```python
from build123d import *

# Parameters (mm, degrees)
F0_W     = 38.1
F0_H     = 25.4
F1_DEPTH = 50.8
F2_D     = 76.2


with BuildPart() as f1:
    # F0 (on Front) → F1 (new body)
    with BuildSketch(Plane.XZ):
        with BuildLine():
            ThreePointArc((0, 103.7758213215), (-54.7329493961, 81.9335598316), (-77.5202206336, 27.5872590731))
            Line((-77.5202206336, 27.5872590731), (-1.3202206336, 27.5872590731))
            Line((-1.3202206336, 27.5872590731), (0, 103.7758213215))
        make_face()
        Polygon((-1.3202206336, 27.5872590731), (-77.5202206336, 27.5872590731), (-77.5202206336, -43.5327409269), (-39.4202206336, -43.5327409269), (36.7797793664, -43.5327409269), (74.8797793664, -43.5327409269), (74.8797793664, 27.5872590731), align=None)
        with BuildLine():
            Line((0, 103.7758213215), (-1.3202206336, 27.5872590731))
            Line((-1.3202206336, 27.5872590731), (74.8797793664, 27.5872590731))
            ThreePointArc((74.8797793664, 27.5872590731), (53.026080125, 80.9999878356), (0, 103.7758213215))
        make_face()
        with Locations((-58.4702206336, -56.2327409269)):
            Rectangle(F0_W, F0_H)
        with Locations((55.8297793664, -56.2327409269)):
            Rectangle(F0_W, F0_H)
    extrude(amount=F1_DEPTH)

    # F2 (through all)
    with Locations(Plane(origin=(0, 0, 0), x_dir=(1, 0, 0), z_dir=(0, 1, 0))):
        with Locations((-1.3202206336, -27.5872590731)):
            Hole(F2_D / 2)


solid = f1.part
```
Could you check a few things on this model? Use its own coordinates, in mm. A direction names the side the tool comes from. Give positions to 0.01 mm unless a question says otherwise; leave off trailing zeros. Loops run counter-clockwise (first coordinate to the right, second up) from the corner with the lowest first, then second, coordinate; pieces in that order, holes last. Notation, with made-up numbers: (6.25, 65) -> (54.25, 65) arc R15 ccw to (54.25, 92) -> close; hole circle Ø4 at (67, -15.5). An arc over 180 degrees is marked (long way). Put each result on its own line as item: value.
(1) Imagine slicing it at D-D on x = 57. Write out the boundary of the cut face in (y, z).
Computed:
outline: (-50.8, -68.93) -> (0, -68.93) -> (0, 76.63) -> (-50.8, 76.63) -> close
(2) Thinking about a two-plate mould opening in X: for faces 3 (the face through (-59, -25, -68.933)), 4 (the face through (-2, -25, -43.533)), 5 (the face through (6.94, -25.76, 64.78)), 6 (the face through (74.88, -25, -21)), which applies, pulls with the +X half, pulls with the -X half, needs draft (parallel to the pull), parting line crosses it, or undercut?
Computed:
face 3: needs draft
face 4: undercut
face 5: undercut
face 6: pulls with the +X half
(3) Imagine slicing it at C-C on z = 63.5. Write out the boundary of the cut face in (x, y), plus the area to 3 significant figures.
Computed:
outline: (-68.53, -50.8) -> (-14.04, -50.8) -> (-14.04, 0) -> (-68.53, 0) -> close; (11.4, -50.8) -> (65.89, -50.8) -> (65.89, 0) -> (11.4, 0) -> close
area: 5,540 mm^2
(4) Imagine slicing it at B-B on x = -37. Write out the boundary of the cut face in (y, z), plus the area to 3 significant figures.
Computed:
outline: (-50.8, -43.53) -> (0, -43.53) -> (0, 14.22) -> (-50.8, 14.22) -> close; (-50.8, 40.95) -> (0, 40.95) -> (0, 94.92) -> (-50.8, 94.92) -> close
area: 5,680 mm^2
(5) Please list where these lines run through material, in increasing order: probe 1 along Z at (x, y) = (-16, -38.5); probe 2 along Z at (x, y) = (20, -16); probe 3 along X at (y, z) = (-7.5, -2). Write a range as [from, to].
Computed:
probe 1: [-43.53, -7.57], [62.75, 102.36]
probe 2: [-43.53, -3.99], [59.16, 100.74]
probe 3: [-77.52, -25.32], [22.68, 74.88]
(6) Imagine slicing it at A-A on y = -41.5. Write out the boundary of the cut face in (x, z).
Computed:
outline: (-77.52, -68.93) -> (-39.42, -68.93) -> (-39.42, -43.53) -> (36.78, -43.53) -> (36.78, -68.93) -> (74.88, -68.93) -> (74.88, 27.59) arc R76.2 ccw to (-77.52, 27.59) -> close; hole circle Ø76.2 at (-1.32, 27.59)
(7) I'm going to push flat-ended pins straight in: pin 1 Ø8 at (y, z) = (-25, 72) entering from +X; pin 2 Ø8 at (x, y) = (46.5, -20.5) entering from +Z. Where does each tip first touch, or does it pass through?
Computed:
pin 1: x = 63.28
pin 2: z = 89.93
(8) For faces 1 (the face through (-77.52, -25, -20)), 2 (the face through (36.78, -25, -56)), which set-ups out of +Z, -Z, +X, -X, +Y, -Y let a thin tool reach every point of the face, with its end or its side?
Computed:
face 1: +Z, -Z, -X, +Y, -Y
face 2: -Z, +Y, -Y
